CAD build for the part. Positions are in the model's coordinates, mm. A direction names the side the tool comes from. Round coordinates to 2 decimals unless told otherwise and drop trailing zeros. Loops run counter-clockwise (first coordinate to the right, second up) from the corner with the lowest first, then second, coordinate; pieces in that order, holes last. Notation, with made-up numbers: M 62,2.5 L 76,2.5 A20 cw 76,27.5 Z; hole C 59,12 d1. An arc over 180 degrees is marked long. Use a Markdown table: item, result. Add a question column.
(1) Band-saw the part on A-A, the plane y = 2. Write the cut outline in (x, z) (3 decimals), and give its area (3 significant figures).
(2) Which spindle directions (+Z, -Z, +X, -X, +Y, -Y) get a long thin tool onto all of the face, cutting with end or side? Do faces 5 (the face through (-92, 3, 6.35)), 6 (the face through (-1, 0, -1)). Say none if no direction does.
(3) Band-saw the part on B-B, the plane z = 0. Write the cut outline in (x, y) (3 decimals), and give its area (3 significant figures).
(4) Two-plate mould, pull along X, no slides. Class faces 1 (the face through (-1, 6.35, -1)), 2 (the face through (86, 3, -31.75)), 3 (the face through (-101.6, 3, 1)), 4 (the face through (101.6, 3, 1)): released by +X, released by -X, zero draft, split by the parting line, or undercut.
(5) Band-saw the part on D-D, the plane z = -22. Write the cut outline in (x, y), and give its area (3 significant figures).
(6) Band-saw the part on C-C, the plane x = -63.5. Write the cut outline in (y, z) (3 decimals).
(7) Wall check: L1, parallel to X at y = 3.5, z = -20.5; L2, parallel to Z at x = -92.5, y = 5 (3 decimals); L3, parallel to X at y = 5, z = 0 (3 decimals). Give the ranges that are in metal, low to high.
from build123d import *

# Parameters (mm, degrees)
SKETCH1_W           = 203.2
SKETCH1_H           = 76.2
SKETCH1_R           = 9.525
SKETCH1_W_2         = 6.35
SKETCH1_H_2         = 15.875
BOSS_EXTRUDE1_DEPTH = 6.35


with BuildPart() as part:
    # Sketch1 → Boss-Extrude1 (new body)
    with BuildSketch(Plane(origin=(0, 0, 0), x_dir=(1, 0, 0), z_dir=(0, 1, 0))):
        Rectangle(SKETCH1_W, SKETCH1_H)
        with Locations(Location((-63.5, 0, 0), (0, 0, 270))):
            Circle(SKETCH1_R, mode=Mode.SUBTRACT)
        with Locations((-92.075, -14.2875)):
            Rectangle(SKETCH1_W_2, SKETCH1_H_2, mode=Mode.SUBTRACT)
        with Locations((-92.075, 23.8125)):
            Rectangle(SKETCH1_W_2, SKETCH1_H_2, mode=Mode.SUBTRACT)
        with Locations((85.725, 23.8125)):
            Rectangle(SKETCH1_W_2, SKETCH1_H_2, mode=Mode.SUBTRACT)
        with Locations((85.725, -14.2875)):
            Rectangle(SKETCH1_W_2, SKETCH1_H_2, mode=Mode.SUBTRACT)
    extrude(amount=BOSS_EXTRUDE1_DEPTH)


solid = part.part
Return value:
| question | item | result |
|---|---|---|
| 1 | outline | M -101.6,-38.1 L 101.6,-38.1 L 101.6,38.1 L -101.6,38.1 Z; hole M -95.25,-31.75 L -88.9,-31.75 L -88.9,-15.875 L -95.25,-15.875 Z; hole M -95.25,6.35 L -88.9,6.35 L -88.9,22.225 L -95.25,22.225 Z; hole C -63.5,0 d19.05; hole M 82.55,-31.75 L 88.9,-31.75 L 88.9,-15.875 L 82.55,-15.875 Z; hole M 82.55,6.35 L 88.9,6.35 L 88.9,22.225 L 82.55,22.225 Z |
| 1 | area | 14,800 mm^2 |
| 2 | face 5 | +Y, -Y |
| 2 | face 6 | +Z, -Z, +X, -X, -Y |
| 3 | outline | M -101.6,0 L -73.025,0 L -73.025,6.35 L -101.6,6.35 Z; M -53.975,0 L 101.6,0 L 101.6,6.35 L -53.975,6.35 Z |
| 3 | area | 1,170 mm^2 |
| 4 | face 1 | zero draft |
| 4 | face 2 | undercut |
| 4 | face 3 | released by -X |
| 4 | face 4 | released by +X |
| 5 | outline | M -101.6,0 L -95.25,0 L -95.25,6.35 L -101.6,6.35 Z; M -88.9,0 L 82.55,0 L 82.55,6.35 L -88.9,6.35 Z; M 88.9,0 L 101.6,0 L 101.6,6.35 L 88.9,6.35 Z |
| 5 | area | 1,210 mm^2 |
| 6 | outline | M 0,-38.1 L 6.35,-38.1 L 6.35,-9.525 L 0,-9.525 Z; M 0,9.525 L 6.35,9.525 L 6.35,38.1 L 0,38.1 Z |
| 7 | L1 | -101.6 to -95.25, -88.9 to 82.55, 88.9 to 101.6 |
| 7 | L2 | -38.1 to -31.75, -15.875 to 6.35, 22.225 to 38.1 |
| 7 | L3 | -101.6 to -73.025, -53.975 to 101.6 |
